from build123d import *

# Parameters (mm, degrees)
TORUS_R                = 0.75
CYLINDER065_R          = 9
CYLINDER065_DEPTH      = 65
CUT094_PLACEMENT_ANGLE = 90


with BuildPart() as torus:
    # Torus → Torus (revolve)
    with BuildSketch(Plane(origin=(0, 0, 60), x_dir=(1, 0, 0), z_dir=(0, -1, 0))):
        with Locations((9.5, 0)):
            Circle(TORUS_R)
    revolve(axis=Axis((0, 0, 60), (0, 0, 1)))


with BuildPart() as cut094:
    # Cylinder065 → Cylinder065 (new body)
    with BuildSketch(Plane.XY):
        Circle(CYLINDER065_R)
    extrude(amount=CYLINDER065_DEPTH)

    # Cut094: cut Torus
    add(torus.part, mode=Mode.SUBTRACT)


with BuildPart() as cut094_1:
    # Cut094 placement: moved
    add(cut094.part.moved(Location((-10, -295, -62))).rotate(Axis((-10, -295, -62), (-1, 0, 0)), CUT094_PLACEMENT_ANGLE))


solid = cut094_1.part
Verification items for the finished model (mm, model axes). Round coordinates to 2 decimals unless told otherwise and drop trailing zeros. Loops run counter-clockwise (first coordinate to the right, second up) from the corner with the lowest first, then second, coordinate; pieces in that order, holes last. Notation, with made-up numbers: (87, 16) - (121, 16) arc R19 ccw to (121, 26) - close; hole circle Ø6 at (50.25, 22). An arc over 180 degrees is marked (long way). Answer in a Markdown table with one row per item. Add a question column.
Q1. Section check A-A on y = -261.5. Enter the section's corners in (x, z), plus the area to 3 significant figures.
Q2. Gauge pin test, flat ends, axial feed: pin 1 (1.5 mm diameter, centred on x = -14.5, y = -278.5, fed in from -Z); pin 2 (2 mm diameter, centred on y = -283, z = -64.5, fed in from +X); pin 3 (5 mm diameter, centred on y = -249.5, z = -66.5, fed in from +X). Record the tip position at first contact, or that the pin passes through.
Q3. Material ranges on line 1 (X direction, y = -263, z = -62.5); line 2 (Z direction, x = -10.25, y = -267.5); line 3 (X direction, y = -269, z = -65), recorded low to high.
Found:
| question | item | result |
|---|---|---|
| 1 | outline | circle Ø18 at (-10, -62) |
| 1 | area | 254 mm² |
| 2 | pin 1 | stops at z = -70.18 |
| 2 | pin 2 | stops at x = -1.13 |
| 2 | pin 3 | stops at x = -1.23 |
| 3 | line 1 | x = -18.99 to -1.01 |
| 3 | line 2 | z = -71 to -53 |
| 3 | line 3 | x = -18.49 to -1.51 |
